Could you check a few things on this model? Use its own coordinates, in mm. A direction names the side the tool comes from. Give positions to 0.01 mm unless a question says otherwise; leave off trailing zeros. Loops run counter-clockwise (first coordinate to the right, second up) from the corner with the lowest first, then second, coordinate; pieces in that order, holes last. Notation, with made-up numbers: M 20,77 L 28,77 A22 cw 28,84 Z; hole C -11,72.25 d1. An arc over 180 degrees is marked long. Answer in a Markdown table with one row per item. Add a question column.
```python
from build123d import *

# Parameters (mm, degrees)
F1_DEPTH = 20
F2_R     = 1
F3_R     = 1.99999


# Not quite as in the source:
# - a fillet or chamfer is up to 0.001 mm smaller than in the source, because OpenCascade refuses the exact size


with BuildPart() as f1:
    # F0 (on Front) → F1 (new body)
    with BuildSketch(Plane.XZ):
        Polygon((-24, 29), (-24, 0), (-20, 0), (-20, 25), (20, 25), (20, -36), (53, -36), (53, 0), (49, 0), (49, -32), (24, -32), (24, 29), align=None)
        with BuildLine():
            Line((-20, 0), (-24, 0))
            ThreePointArc((-24, 0), (-20.3284271247, -3.8639610307), (-15, -4))
            Line((-15, -4), (-15, 0))
            Line((-15, 0), (-20, 0))
        make_face()
    extrude(amount=F1_DEPTH)

    # F2
    f2_edges = [f1.edges().sort_by_distance(p)[0] for p in [
        (-20, -10, 0),
        (-20, -10, 25),
        (20, -10, 25),
        (24, -10, -32),
        (49, -10, -32),
    ]]
    fillet(f2_edges, radius=F2_R)

    # F3 (radius 2 in the source; OpenCascade refuses exactly that, so slightly less here)
    f3_edges = [f1.edges().sort_by_distance(p)[0] for p in [
        (-24, -10, 29),
        (24, -10, 29),
        (20, -10, -36),
        (53, -10, -36),
        (49, -10, 0),
        (53, -10, 0),
    ]]
    fillet(f3_edges, radius=F3_R)


solid = f1.part
```
Item 1: For faces 1 (the face through (-24, -10, 14)), 2 (the face through (49.6, -10.14, -0.57)), 3 (the face through (20, -10, -5)), which set-ups out of +Z, -Z, +X, -X, +Y, -Y let a thin tool reach every point of the face, with its end or its side?
Item 2: For P1, Ø10, axis at x = 32.5, z = 4.5, coming from the -Y side; P2, Ø10, axis at y = -11.5, z = 7.5, coming from the +X side; P3, Ø5, axis at x = 33, y = -2.5, coming from the +Z side; P4, Ø1.5, axis at y = -9, z = -20.5, coming from the -X side, each with a flat end and sliding along its axis, tell me the tip position at first contact or that it passes through.
Item 3: Suppose I cut it at B-B (x = -17.5). List the corners of the cut face in (y, z) for me.
Item 4: I need wall thicknesses on L1, parallel to X at y = -2, z = -4.5; L2, parallel to X at y = -17, z = -3; L3, parallel to X at y = -4, z = 3. Which ranges of each line are inside material? Lowest first, please.
Item 5: Suppose I cut it at A-A (z = 15). List the corners of the cut face in (x, y) for me, then the cut area to 3 significant figures.
Item 6: If we mould it in two halves opening along Z, with no side actions, what happens to faces 4 (the face through (-20, -10, 12)), 5 (the face through (37, -10, -32)), 6 (the face through (-17, -10, 0)), 7 (the face through (24, -10, -2))? For each: +Z half, -Z half, draft (parallel to the pull), parting line (faces both ways), or undercut.
Item 7: Suppose I cut it at D-D (x = 6.5). List the corners of the cut face in (y, z) for me.
Values found:
| question | item | result |
|---|---|---|
| 1 | face 1 | +Z, -Z, -X, +Y, -Y |
| 1 | face 2 | +Z, +Y, -Y |
| 1 | face 3 | -Z, +Y, -Y |
| 2 | P1 | through |
| 2 | P2 | x = 24 |
| 2 | P3 | z = -32 |
| 2 | P4 | x = 20 |
| 3 | outline | M -20,-4.46 L 0,-4.46 L 0,0 L -20,0 Z; M -20,25 L 0,25 L 0,29 L -20,29 Z |
| 4 | L1 | 20 to 24, 49 to 53 |
| 4 | L2 | -21.77 to -15, 20 to 24, 49 to 53 |
| 4 | L3 | -24 to -20, 20 to 24 |
| 5 | outline | M -24,-20 L -20,-20 L -20,0 L -24,0 Z; M 20,-20 L 24,-20 L 24,0 L 20,0 Z |
| 5 | area | 160 mm² |
| 6 | face 4 | undercut |
| 6 | face 5 | +Z half |
| 6 | face 6 | undercut |
| 6 | face 7 | draft |
| 7 | outline | M -20,25 L 0,25 L 0,29 L -20,29 Z |
